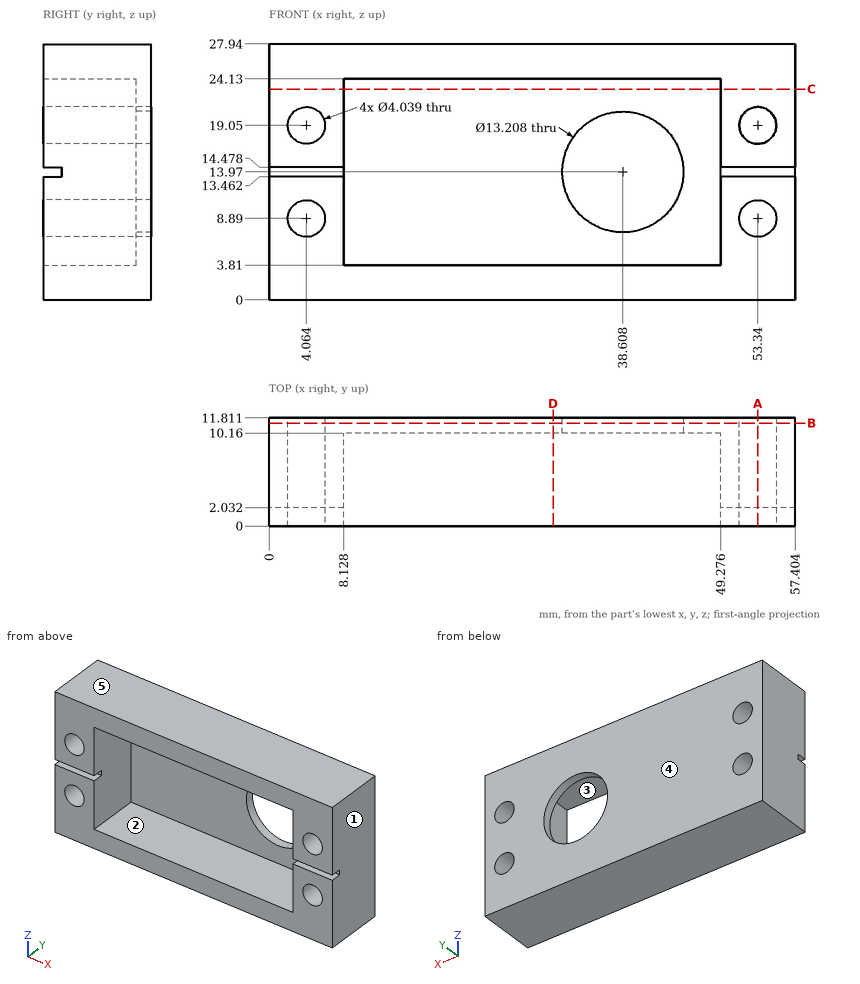
Geometry check sheet. Reference: drawing and pictorial views, mm from the part's lowest x, y, z. A direction names the side the tool comes from. Round coordinates to 2 decimals unless told otherwise and drop trailing zeros. Order: outer loops, then holes, each group sorted by start corner. A loop starts at its lowest first (then second) coordinate and runs counter-clockwise, first axis right, second up. Notation, with made-up numbers: M 39.5,75.25 L 61.5,75.25 A28 ccw 61.5,94.25 Z; hole C 68,43 d6. An arc over 180 degrees is marked long. Answer in a Markdown table with one row per item.
(1) Sectioned sample at B-B, the plane y = 11.25. State how many separate pieces and enclosed holes the cut face has, and give its area (3 significant figures).
Responses:
| item | result |
|---|---|
| separate pieces | 1 |
| enclosed holes | 5 |
| area | 1,420 mm² |
(2) Sectioned sample at D-D, the plane x = 31. Record the cut outline in (y, z).
Responses:
| item | result |
|---|---|
| outline | M 0,0 L 11.81,0 L 11.81,27.94 L 0,27.94 L 0,24.13 L 10.16,24.13 L 10.16,3.81 L 0,3.81 Z |
(3) Sectioned sample at A-A, the plane x = 53.34. Record the cut outline in (y, z).
Responses:
| item | result |
|---|---|
| outline | M 0,0 L 11.81,0 L 11.81,6.87 L 0,6.87 Z; M 0,10.91 L 11.81,10.91 L 11.81,17.03 L 0,17.03 L 0,14.48 L 2.03,14.48 L 2.03,13.46 L 0,13.46 Z; M 0,21.07 L 11.81,21.07 L 11.81,27.94 L 0,27.94 Z |
(4) Scan lines: probe 1 along Z at (x, y) = (4, 3); probe 2 along Z at (x, y) = (45.5, 6.25); probe 3 along Z at (x, y) = (54, 4.5). Record each from-to range of solid material in increasing order. Write a range as from..to.
Responses:
| item | result |
|---|---|
| probe 1 | z = 0..6.87, 10.91..17.03, 21.07..27.94 |
| probe 2 | z = 0..3.81, 24.13..27.94 |
| probe 3 | z = 0..6.98, 10.8..17.14, 20.96..27.94 |
(5) Sectioned sample at C-C, the plane z = 23. Record the cut outline in (x, y).
Responses:
| item | result |
|---|---|
| outline | M 0,0 L 8.13,0 L 8.13,10.16 L 49.28,10.16 L 49.28,0 L 57.4,0 L 57.4,11.81 L 0,11.81 Z |
(6) Draft check along Z on the marked faces 3, 4 and 5. Enter one of: released by +Z, released by -Z, zero draft, split by the parting line, or undercut.
Responses:
| item | result |
|---|---|
| face 3 | undercut |
| face 4 | zero draft |
| face 5 | released by +Z |
(7) Tool access check on the marked faces 1 and 2. Record the directions out of +Z, -Z, +X, -X, +Y, -Y that give a thin tool (end or side, any length) a straight path to the whole face; none if there is none.
Responses:
| item | result |
|---|---|
| face 1 | +Z, -Z, +X, +Y, -Y |
| face 2 | -Y |
(8) Go/stop test with flat-tipped pins: P1, Ø2.5, axis at x = 53.34, z = 8.89, coming from the +Y side; P2, Ø6, axis at x = 19.5, z = 16.5, coming from the -Y side. Record where each tip stops, or that it passes through.
Responses:
| item | result |
|---|---|
| P1 | passes through |
| P2 | stops at y = 10.16 |
